```python
from build123d import *

# Parameters (mm, degrees)
F0_W     = 38.1
F0_H     = 914.4
F1_DEPTH = 88.9
F3_DEPTH = 88.9
F5_DEPTH = 88.9


with BuildPart() as f1:
    # F0 (on Front) → F1 (new body)
    with BuildSketch(Plane.XZ):
        with Locations((-19.05, 457.2)):
            Rectangle(F0_W, F0_H)
    extrude(amount=F1_DEPTH)

    # F2 (on face) → F3 (cut)
    with BuildSketch(Plane.XZ.offset(88.9)):
        Polygon((0, 914.4), (-38.1, 914.4), (0, 900.532734), align=None)
    extrude(amount=-F3_DEPTH, mode=Mode.SUBTRACT)

    # F4 (on face) → F5 (cut)
    with BuildSketch(Plane.XZ.offset(88.9)):
        Polygon((-38.1, 0), (0, 0), (-38.1, 13.867266), align=None)
    extrude(amount=-F5_DEPTH, mode=Mode.SUBTRACT)


solid = f1.part
```
For this review, take the finished solid that the model builds, in its own axes (mm). Round coordinates to 2 decimals unless told otherwise and drop trailing zeros. Order: outer loops, then holes, each group sorted by start corner. A loop starts at its lowest first (then second) coordinate and runs counter-clockwise, first axis right, second up. Notation, with made-up numbers: (21.5, 85.5) -> (74.5, 85.5) arc R19 ccw to (74.5, 102.5) -> close; hole circle Ø1 at (-1, 59.5). An arc over 180 degrees is marked (long way). Use a Markdown table: item, result.
Item 1: For line 1 along Z through (x, y) = (-8.5, -36.5); line 2 along Z through (x, y) = (-7, -72), list the stretches that pass through material, from the lowest coordinate up. Write a range as [from, to].
Resolved:
| item | result |
|---|---|
| line 1 | z = [3.09, 903.63] |
| line 2 | z = [2.55, 903.08] |
Item 2: For pin 1 (5 mm diameter, centred on x = -11.5, z = 694.5, fed in from +Y); pin 2 (12 mm diameter, centred on x = -30, y = -32, fed in from +Z); pin 3 (12 mm diameter, centred on x = -19, y = -48, fed in from -Z); pin 4 (1 mm diameter, centred on x = -5.5, y = -69.5, fed in from -Z), all flat-tipped, find the tip position at first contact; note any pin that passes through.
Resolved:
| item | result |
|---|---|
| pin 1 | stops at y = 0 |
| pin 2 | stops at z = 913.64 |
| pin 3 | stops at z = 4.73 |
| pin 4 | stops at z = 1.82 |
Item 3: Take a section at B-B (x = -19). State the section outline as (y, z) points.
Resolved:
| item | result |
|---|---|
| outline | (-88.9, 6.92) -> (0, 6.92) -> (0, 907.45) -> (-88.9, 907.45) -> close |
Item 4: Take a section at A-A (y = -63.5). State the section outline as (x, z) points, plus the area to 3 significant figures.
Resolved:
| item | result |
|---|---|
| outline | (-38.1, 13.87) -> (0, 0) -> (0, 900.53) -> (-38.1, 914.4) -> close |
| area | 34,300 mm² |
